Geometry: final body of the model. Coordinates: model frame, mm. A direction names the side the tool comes from. Give positions to 0.01 mm unless a question says otherwise; leave off trailing zeros. Order: outer loops, then holes, each group sorted by start corner. A loop starts at its lowest first (then second) coordinate and runs counter-clockwise, first axis right, second up. Notation, with made-up numbers: (5.25, 10) -> (47.25, 10) arc R22 ccw to (47.25, 37) -> close; hole circle Ø4 at (59, -20.5). An arc over 180 degrees is marked (long way). Write item = value, one per line.
Autodesk Inventor part; units mm, degrees
ref_plane "YZ Plane" through (0, 0, 0) normal (1, 0, 0) x (0, 1, 0)
ref_plane "XZ Plane" through (0, 0, 0) normal (0, 1, 0) x (-1, 0, 0)
ref_plane "XY Plane" through (0, 0, 0) normal (0, 0, 1) x (1, 0, 0)
sketch "스케치1" plane through (0, 0, 0) normal (0, 1, 0) x (-1, 0, 0)
  circle A0 centre (0, 0) radius 30
  circle A1 centre (0, 0) radius 10
  dimension "d0" = 60
  dimension "d1" = 20
extrude "돌출1" add sketch "스케치1" along normal blind 5
extrude "돌출2" add sketch "스케치1" along normal blind 250 contours A1
sketch "스케치2" plane through (0, 250, 0) normal (0, 1, 0) x (1, 0, 0)
  circle A0 centre (0, 0) radius 25
  dimension "d6" = 50
extrude "돌출3" add sketch "스케치2" along normal blind 80
sketch "스케치6" plane through (0, 330, 0) normal (0, 1, 0) x (1, 0, 0)
  circle A0 centre (0, 0) radius 25
  circle A1 centre (0, 0) radius 24
  dimension "d15" = 48
extrude "돌출6" add sketch "스케치6" along normal blind 30 contours A1
sketch "스케치7" plane through (0, 360, 0) normal (0, 1, 0) x (1, 0, 0)
  circle A0 centre (0, 0) radius 25
  dimension "d18" = 50
extrude "돌출7" add sketch "스케치7" along normal blind 5
sketch "스케치8" plane through (0, 365, 0) normal (0, 1, 0) x (1, 0, 0)
  circle A0 centre (0, 0) radius 24
  dimension "d21" = 48
extrude "돌출8" add sketch "스케치8" along normal blind 30
sketch "스케치9" plane through (0, 395, 0) normal (0, 1, 0) x (1, 0, 0)
  circle A0 centre (0, 0) radius 25
  dimension "d24" = 50
extrude "돌출9" add sketch "스케치9" along normal blind 20
properties part number "led"
1) Reachability of faces 4 (the face through (0, 250, 11)), 5 (the face through (23.846, 362.465, 7.509)), 6 (the face through (0, 0, 0)) from +Z, -Z, +X, -X, +Y, -Y: full face, straight path, thin tool, end or side. Return the list, or none.
Check sheet entries:
face_4 = none
face_5 = +Y
face_6 = +Z, -Z, +X, -X, -Y
2) Mould query, pull axis Y, two halves, no side actions, for faces 1 (the face through (0, 415, 0)), 2 (the face through (-23.977, 344.79, 1.055)), 3 (the face through (29.97, 2.46, -1.32)). Classes: +Y half, -Y half, draft (parallel to the pull), parting line (faces both ways), or undercut.
Check sheet entries:
face_1 = +Y half
face_2 = undercut
face_3 = draft
3) Section query B-B (z = -17.5). Output: boundary loops of the cut face in (x, y), plus the area to 3 significant figures.
Check sheet entries:
outline = (-24.37, 0) -> (24.37, 0) -> (24.37, 5) -> (-24.37, 5) -> close; (-17.85, 250) -> (17.85, 250) -> (17.85, 330) -> (16.42, 330) -> (16.42, 360) -> (17.85, 360) -> (17.85, 365) -> (16.42, 365) -> (16.42, 395) -> (17.85, 395) -> (17.85, 415) -> (-17.85, 415) -> (-17.85, 395) -> (-16.42, 395) -> (-16.42, 365) -> (-17.85, 365) -> (-17.85, 360) -> (-16.42, 360) -> (-16.42, 330) -> (-17.85, 330) -> close
area = 5,960 mm²
4) Section query A-A (x = 0). Output: boundary loops of the cut face in (y, z).
Check sheet entries:
outline = (0, -30) -> (5, -30) -> (5, -10) -> (250, -10) -> (250, -25) -> (330, -25) -> (330, -24) -> (360, -24) -> (360, -25) -> (365, -25) -> (365, -24) -> (395, -24) -> (395, -25) -> (415, -25) -> (415, 25) -> (395, 25) -> (395, 24) -> (365, 24) -> (365, 25) -> (360, 25) -> (360, 24) -> (330, 24) -> (330, 25) -> (250, 25) -> (250, 10) -> (5, 10) -> (5, 30) -> (0, 30) -> close
5) First-contact query: P1, Ø10, axis at x = 11, y = 334.5, coming from the +Z side; P2, Ø1, axis at y = 262.5, z = -8, coming from the -X side; P3, Ø1.5, axis at x = 21, y = 264.5, coming from the +Z side. Flat tips, straight axial feed; report the tip coordinate or a pass-through.
Check sheet entries:
P1 = 23.39
P2 = -23.85
P3 = 14.66
6) Section query C-C (z = 0). Output: boundary loops of the cut face in (x, y), plus the area to 3 significant figures.
Check sheet entries:
outline = (-30, 0) -> (30, 0) -> (30, 5) -> (10, 5) -> (10, 250) -> (25, 250) -> (25, 330) -> (24, 330) -> (24, 360) -> (25, 360) -> (25, 365) -> (24, 365) -> (24, 395) -> (25, 395) -> (25, 415) -> (-25, 415) -> (-25, 395) -> (-24, 395) -> (-24, 365) -> (-25, 365) -> (-25, 360) -> (-24, 360) -> (-24, 330) -> (-25, 330) -> (-25, 250) -> (-10, 250) -> (-10, 5) -> (-30, 5) -> close
area = 13,300 mm²
7) Line query: line 1 (Y direction, x = 22, z = -11); line 2 (Y direction, x = 18, z = -4.5); line 3 (Y direction, x = 26.5, z = 3.5). Output: solid intervals per line, ascending. Write a range as from..to.
Check sheet entries:
line_1 = 0..5, 250..330, 360..365, 395..415
line_2 = 0..5, 250..415
line_3 = 0..5
8) Section query D-D (y = 163). Output: boundary loops of the cut face in (x, z), plus the area to 3 significant figures.
Check sheet entries:
outline = circle Ø20 at (0, 0)
area = 314 mm²
